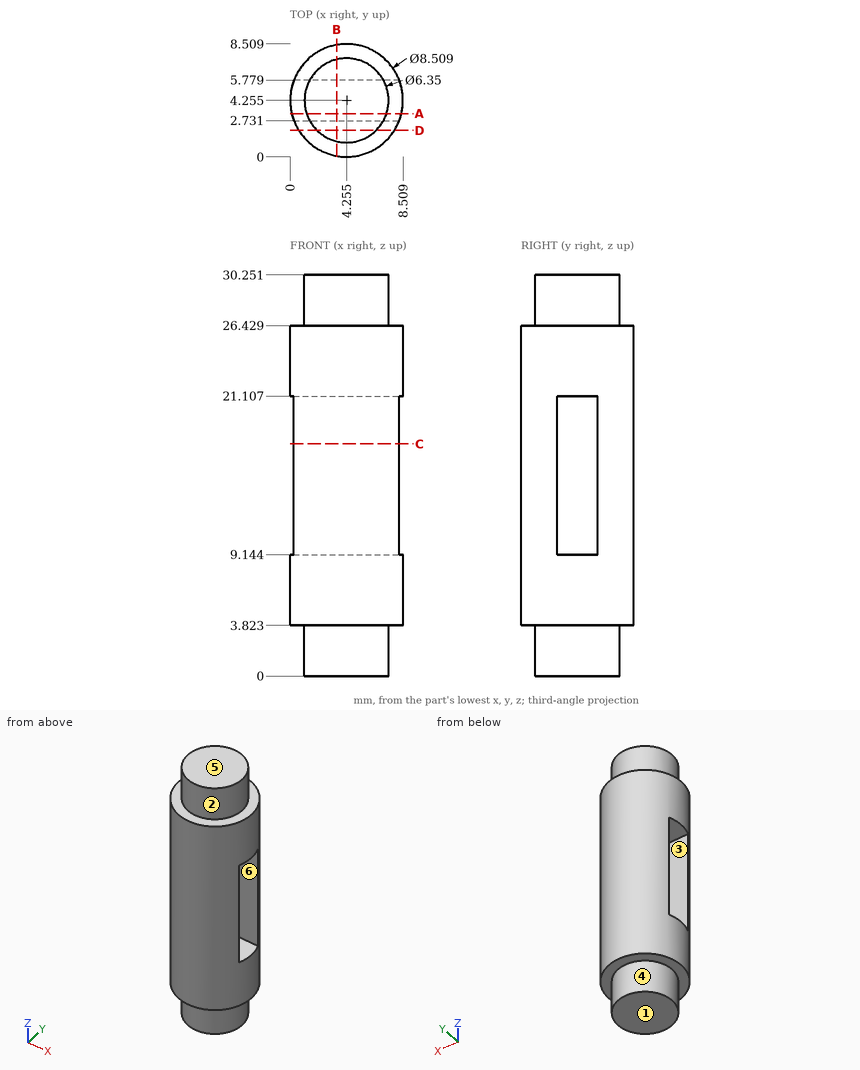
Design review of the part shown in the three views and the two pictorial views. Dimensions are in mm from the part's minimum x, y and z. A direction names the side the tool comes from. Round coordinates to 2 decimals unless told otherwise and drop trailing zeros. Write each loop counter-clockwise with the first axis right and the second up, starting at its lowest first coordinate (ties: lowest second). Pieces come first, ordered by that corner, then holes. Notation, with made-up numbers: M 87.25,10.5 L 121.25,10.5 A19 ccw 121.25,45.5 Z; hole C 55.25,52 d4. An arc over 180 degrees is marked long. Use a Markdown table: item, result. Add a question column.
Q1. The part is to be moulded in two halves that separate along Z. For the marked faces 1, 2 and 3, say which applies: pulls with the +Z half, pulls with the -Z half, needs draft (parallel to the pull), parting line crosses it, or undercut.
Q2. Insertion check: pin 1 (1 mm diameter, centred on x = 1, z = 19.5, fed in from -Y); pin 2 (3 mm diameter, centred on y = 2, z = 27, fed in from +X); pin 3 (2 mm diameter, centred on x = 2, z = 20.5, fed in from -Y). Each pin has a flat end and moves straight along its axis. Give the tip position at first contact, or say it passes through.
Q3. We need section D-D, the plane y = 2. State the section outline as (x, z) points.
Q4. We need section C-C, the plane z = 17.5. State the section outline as (x, y) points (1 decimal).
Q5. We need section A-A, the plane y = 3.25. State the section outline as (x, z) points (1 decimal), plus the area to 3 significant figures.
Q6. Machinability: for the marked faces 4, 5 and 6, which of the approach directions +Z, -Z, +X, -X, +Y, -Y give a long, thin tool a straight path to every point of the face, cutting with its end or side? Answer none if there is none.
Q7. We need section B-B, the plane x = 3.5. State the section outline as (y, z) points (1 decimal).
Q8. To check wall thickness, follow line 1 (Z direction, x = 7.75, y = 5) (1 decimal); line 2 (Z direction, x = 7, y = 3.5) (1 decimal); line 3 (Y direction, x = 1, z = 20) (1 decimal). State the ranges of each line that lie inside material, in increasing order.
Findings below:
| question | item | result |
|---|---|---|
| 1 | face 1 | pulls with the -Z half |
| 1 | face 2 | needs draft |
| 1 | face 3 | undercut |
| 2 | pin 1 | stops at y = 1.01 |
| 2 | pin 2 | stops at x = 8.42 |
| 2 | pin 3 | stops at y = 0.19 |
| 3 | outline | M 0.65,3.82 L 2.02,3.82 L 2.02,0 L 6.49,0 L 6.49,3.82 L 7.86,3.82 L 7.86,26.43 L 6.49,26.43 L 6.49,30.25 L 2.02,30.25 L 2.02,26.43 L 0.65,26.43 Z |
| 4 | outline | M 0.3,2.7 A4.3 ccw 8.2,2.7 Z; M 0.3,5.8 L 8.2,5.8 A4.3 ccw Z |
| 5 | outline | M 0.1,3.8 L 1.2,3.8 L 1.2,0 L 7.3,0 L 7.3,3.8 L 8.4,3.8 L 8.4,9.1 L 0.1,9.1 Z; M 0.1,21.1 L 8.4,21.1 L 8.4,26.4 L 7.3,26.4 L 7.3,30.3 L 1.2,30.3 L 1.2,26.4 L 0.1,26.4 Z |
| 5 | area | 134 mm² |
| 6 | face 4 | -Z |
| 6 | face 5 | +Z, +X, -X, +Y, -Y |
| 6 | face 6 | +X, -X |
| 7 | outline | M 0.1,3.8 L 1.2,3.8 L 1.2,0 L 7.3,0 L 7.3,3.8 L 8.4,3.8 L 8.4,26.4 L 7.3,26.4 L 7.3,30.3 L 1.2,30.3 L 1.2,26.4 L 0.1,26.4 Z; hole M 2.7,9.1 L 5.8,9.1 L 5.8,21.1 L 2.7,21.1 Z |
| 8 | line 1 | z = 3.8 to 9.1, 21.1 to 26.4 |
| 8 | line 2 | z = 0 to 9.1, 21.1 to 30.3 |
| 8 | line 3 | y = 1.5 to 2.7, 5.8 to 7 |
